Autodesk Inventor part; units mm, degrees
ref_plane "cp1_XY" through (33.8074, 6.1468, 0) normal (1, 0, 0) x (0, 0, -1)
ref_plane "cp1_YZ" through (33.8074, 6.1468, 0) normal (0, 0, -1) x (0, 1, 0)
ref_plane "cp1_ZX" through (33.8074, 6.1468, 0) normal (0, 1, 0) x (1, 0, 0)
sketch "Sketch_1" plane through (0, 0, 0) normal (0, 0, 1) x (1, 0, 0)
  line L0 (67.6148, 0) -> (0, 0)
  arc A0 (-0.3964, 5.4846) -> (-0.3964, 5.305) centre (-0.3066, 5.3948) ccw
  line L1 (-0.3964, 5.305) -> (-0.254, 5.1626)
  line L2 (-0.254, 5.1626) -> (0, 5.1626)
  line L3 (0, 5.1626) -> (0.508, 5.6706)
  line L4 (0.508, 5.6706) -> (67.1068, 5.6706)
  line L5 (67.1068, 5.6706) -> (67.6148, 5.1626)
  line L6 (67.6148, 5.1626) -> (67.8688, 5.1626)
  line L7 (67.8688, 5.1626) -> (68.0112, 5.305)
  arc A1 (68.0112, 5.305) -> (68.0112, 5.4846) centre (67.9214, 5.3948) ccw
  line L8 (68.0112, 5.4846) -> (67.4978, 5.998)
  arc A2 (67.4978, 5.998) -> (67.1385, 6.1468) centre (67.1385, 5.6388) ccw
  line L9 (67.1385, 6.1468) -> (0.4763, 6.1468)
  arc A3 (0.4763, 6.1468) -> (0.117, 5.998) centre (0.4763, 5.6388) ccw
  line L10 (0.117, 5.998) -> (-0.3964, 5.4846)
revolve "Revolution1" add sketch "Sketch_1" angle 360 about axis through (67.6148, 0, 0) along (1, 0, 0)
sketch "Sketch_4" plane through (0, 0, 0) normal (0, 0, 1) x (1, 0, 0)
  circle A0 centre (5.842, 0) radius 0.7874
extrude "Extrusion1" cut sketch "Sketch_4" along normal blind 6.1468
ref_plane "cp1_XY" through (33.8074, 6.1468, 0) normal (1, 0, 0) x (0, 0, -1)
ref_plane "cp1_YZ" through (33.8074, 6.1468, 0) normal (0, 0, -1) x (0, 1, 0)
ref_plane "cp1_ZX" through (33.8074, 6.1468, 0) normal (0, 1, 0) x (1, 0, 0)
ref_plane "cp2_XY" through (33.8074, 0, -6.1468) normal (1, 0, 0) x (0, 0, -1)
ref_plane "cp2_YZ" through (33.8074, 0, -6.1468) normal (0, 0, -1) x (0, 1, 0)
ref_plane "cp2_ZX" through (33.8074, 0, -6.1468) normal (0, 1, 0) x (1, 0, 0)
ref_plane "cp3_XY" through (33.8074, -6.1468, 0) normal (1, 0, 0) x (0, 0, -1)
ref_plane "cp3_YZ" through (33.8074, -6.1468, 0) normal (0, 0, -1) x (0, 1, 0)
ref_plane "cp3_ZX" through (33.8074, -6.1468, 0) normal (0, 1, 0) x (1, 0, 0)
ref_plane "cp4_XY" through (33.8074, 0, 6.1468) normal (1, 0, 0) x (0, 0, -1)
ref_plane "cp4_YZ" through (33.8074, 0, 6.1468) normal (0, 0, -1) x (0, 1, 0)
ref_plane "cp4_ZX" through (33.8074, 0, 6.1468) normal (0, 1, 0) x (1, 0, 0)
ref_plane "tube_front_XY" through (0, 0, 0) normal (1, 0, 0) x (0, 0, -1)
ref_plane "tube_front_YZ" through (0, 0, 0) normal (0, 0, -1) x (0, 1, 0)
ref_plane "tube_front_ZX" through (0, 0, 0) normal (0, 1, 0) x (1, 0, 0)
ref_plane "tube_rear_XY" through (67.6148, 0, 0) normal (1, 0, 0) x (0, 0, -1)
ref_plane "tube_rear_YZ" through (67.6148, 0, 0) normal (0, 0, -1) x (0, 1, 0)
ref_plane "tube_rear_ZX" through (67.6148, 0, 0) normal (0, 1, 0) x (1, 0, 0)
properties part number "01-2.6622"
Build history of the part. All positions in model axes, mm. A direction names the side the tool comes from. Coordinates: 2 decimals unless noted, no trailing zeros. Order: outer loops, then holes, each group sorted by start corner. A loop starts at its lowest first (then second) coordinate and runs counter-clockwise, first axis right, second up. Notation, with made-up numbers: (-28, 58.25) - (13, 58.25) arc R20 ccw to (13, 79.25) - close; hole circle Ø8 at (53.25, -26.5). An arc over 180 degrees is marked (long way). Write item = value, one per line. Start each with the question number.
1) Saw through at C-C on x = 54. Write the cut outline in (y, z).
2) Flat gauge pins, fed straight in: pin 1 Ø1.5 at (y, z) = (2, -3) entering from -X (3 decimals); pin 2 Ø4 at (x, y) = (7.5, -4.5) entering from +Z. Where does each tip first touch, or does it go through?
3) Saw through at D-D on x = 6. Write the cut outline in (y, z).
4) 3-axis set-ups, long thin cutter, end or side, ignore diameter. For faces 1 (the face through (5.055, -0.035, 5.878)), 2 (the face through (34.27, 2.62, -5.03)), 3 (the face through (33.34, 5.86, -1.85)): which of +Z, -Z, +X, -X, +Y, -Y reach the whole face in a straight line?
5) Saw through at A-A on y = 0. Count the separate pieces of the cut face and the enclosed holes in it, then the cut area to 3 significant figures.
6) Wall check: line 1 along Y through (x, z) = (30, -0.25); line 2 along Y through (x, z) = (45, 3.5); line 3 along Z through (x, y) = (29, 1). Give the ranges that are in metal, low to high. Write a range as from..to.
From the geometry:
q1.outline = circle Ø12.29 at (0, 0); hole circle Ø11.34 at (0, 0)
q2.pin_1 = through
q2.pin_2 = 5.62
q3.outline = (-0.77, 5.62) - (-0.77, 6.1) arc R6.15 ccw (long way) to (0.77, 6.1) - (0.77, 5.62) arc R5.67 cw (long way) to start
q4.face_1 = +Z
q4.face_2 = none
q4.face_3 = +X, -X
q5.separate_pieces = 3
q5.enclosed_holes = 0
q5.area = 64.8 mm^2
q6.line_1 = -6.14..-5.67, 5.67..6.14
q6.line_2 = -5.05..-4.46, 4.46..5.05
q6.line_3 = -6.06..-5.58, 5.58..6.06
